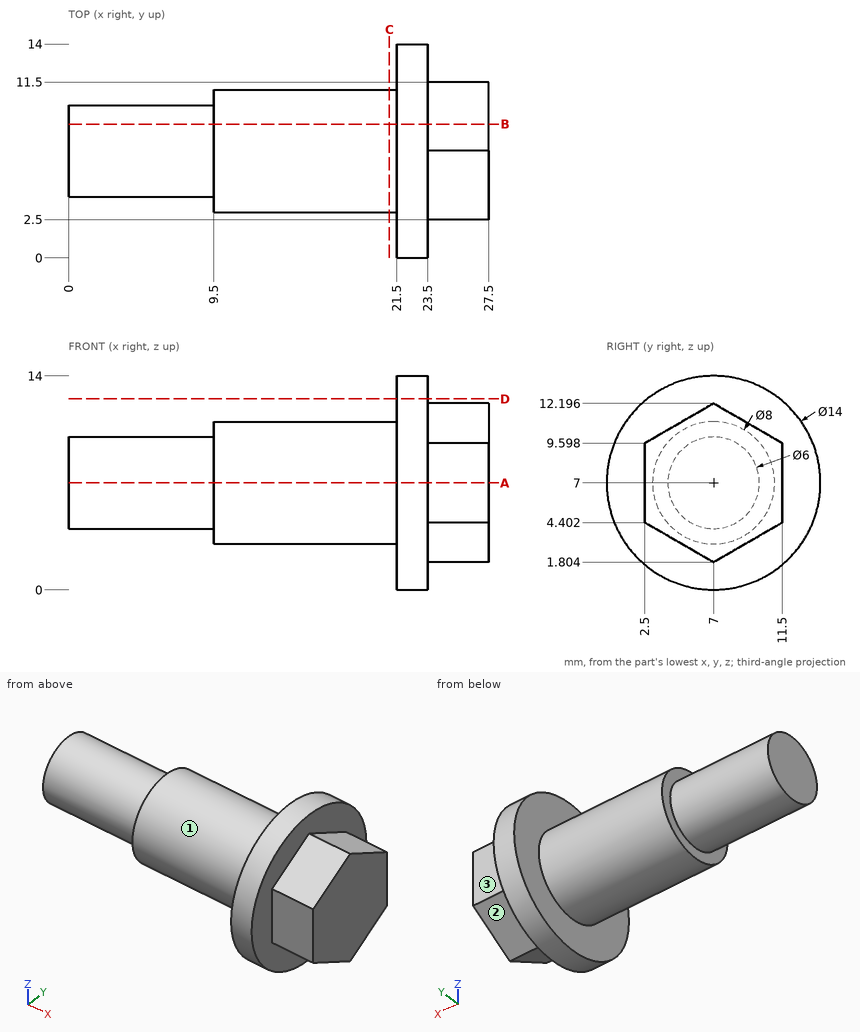
Verification items for this drawing (mm, ordinates from the low corner). A direction names the side the tool comes from. Round coordinates to 2 decimals unless told otherwise and drop trailing zeros. Loops run counter-clockwise (first coordinate to the right, second up) from the corner with the lowest first, then second, coordinate; pieces in that order, holes last. Notation, with made-up numbers: (-31, 64) - (18, 64) arc R26 cw to (18, 81) - close; hole circle Ø6 at (31, 25). An arc over 180 degrees is marked (long way). Answer as CSV lines item,"result". Start each with the question number.
Item 1: Section check A-A (z = 7). Record the boundary of the cut face in (x, y).
Item 2: Scan lines: line 1 (X direction, y = 2.25, z = 5.5); line 2 (X direction, y = 8.5, z = 11); line 3 (Z direction, x = 8.5, y = 8.5). Record each from-to range of solid material in increasing order. Write a range as [from, to].
Item 3: Section check D-D (z = 12.5). Record the boundary of the cut face in (x, y).
Item 4: Depth check by flat-ended pin: P1, Ø1, axis at x = 23, y = 5.5, coming from the +Z side; P2, Ø4.5, axis at x = 26.5, z = 6, coming from the +Y side; P3, Ø2, axis at x = 13.5, z = 2.5, coming from the +Y side. Enter the tip coordinate at first touch or a pass-through.
Item 5: Section check B-B (y = 8.75). Record the boundary of the cut face in (x, z), and give its area (3 significant figures).
Item 6: Section check C-C (x = 21). Record the boundary of the cut face in (y, z), and give its area (3 significant figures).
Item 7: Set-up check for the marked faces 1, 2 and 3: record each of +Z, -Z, +X, -X, +Y, -Y from which the full face is reachable in a straight line by a thin tool's end or side.
Report:
1,outline,"(0, 4) - (9.5, 4) - (9.5, 3) - (21.5, 3) - (21.5, 0) - (23.5, 0) - (23.5, 2.5) - (27.5, 2.5) - (27.5, 11.5) - (23.5, 11.5) - (23.5, 14) - (21.5, 14) - (21.5, 11) - (9.5, 11) - (9.5, 10) - (0, 10) - close"
2,line 1,"x = [21.5, 23.5]"
2,line 2,"x = [21.5, 27.5]"
2,line 3,"z = [4.4, 9.6]"
3,outline,"(21.5, 2.67) - (23.5, 2.67) - (23.5, 11.33) - (21.5, 11.33) - close"
4,P1,"stops at z = 13.93"
4,P2,"stops at y = 11.5"
4,P3,"stops at y = 8.94"
5,outline,"(0, 4.56) - (9.5, 4.56) - (9.5, 3.4) - (21.5, 3.4) - (21.5, 0.22) - (23.5, 0.22) - (23.5, 2.81) - (27.5, 2.81) - (27.5, 11.19) - (23.5, 11.19) - (23.5, 13.78) - (21.5, 13.78) - (21.5, 10.6) - (9.5, 10.6) - (9.5, 9.44) - (0, 9.44) - close"
5,area,"193 mm2"
6,outline,"circle Ø8 at (7, 7)"
6,area,"50.3 mm2"
7,face 1,"-X"
7,face 2,"-Z, +X, +Y"
7,face 3,"+Z, -Z, +X, +Y"
